Autodesk Inventor part; units mm, degrees
ref_plane "YZ Plane" through (0, 0, 0) normal (1, 0, 0) x (0, 1, 0)
ref_plane "XZ Plane" through (0, 0, 0) normal (0, 1, 0) x (-1, 0, 0)
ref_plane "XY Plane" through (0, 0, 0) normal (0, 0, 1) x (1, 0, 0)
sketch "Sketch1" plane through (0, 0, 0) normal (0, 1, 0) x (-1, 0, 0)
  line L0 (-13, 22.45) -> (13, 22.45)
  line L1 (13, 22.45) -> (13, -22.45)
  line L2 (13, -22.45) -> (-13, -22.45)
  line L3 (-13, -22.45) -> (-13, 22.45)
  line L4 (-13, 22.45) -> (13, -22.45) construction
  line L5 (13, 22.45) -> (-13, -22.45) construction
  point P0 (0, 0)
  dimension "d0" = 26
  dimension "d1" = 44.9
extrude "Extrusion1" add sketch "Sketch1" along normal blind 50
sketch "Sketch2" plane through (-13, 0, 22.45) normal (0, 0, 1) x (1, 0, 0)
  line L0 (0, 0) -> (26, 0)
  line L1 (26, 0) -> (26, 50)
  line L2 (0, 50) -> (26, 50)
  line L3 (0, 0) -> (0, 50)
  line L4 (13, 50) -> (13, 0)
  line L5 (13, 50) -> (7, 50)
  line L6 (26, 50) -> (0, 50)
  line L7 (7, 50) -> (7, 31)
  line L8 (7, 31) -> (19, 31)
  line L9 (19, 31) -> (19, 50)
  line L10 (13, 50) -> (19, 50)
  dimension "d4" = 6
  dimension "d5" = 19
  dimension "d6" = 12
extrude "Extrusion2" cut sketch "Sketch2" against normal blind 50 contours L8 L7 L2 L4 | L4 L2 L9 L8
sketch "Sketch3" plane through (13, 0, 22.45) normal (1, 0, 0) x (0, 0, -1)
  circle A0 centre (7.35, 39.4) radius 1.9
  circle A1 centre (37.55, 39.4) radius 1.9
  line L0 (0, 50) -> (44.9, 50)
  line L1 (22.45, 50) -> (22.45, 0)
  line L2 (44.9, 0) -> (0, 0)
  point P0 (22.45, 25)
  point P1 (3.8014, 50)
  dimension "d9" = 3.8
extrude "Extrusion3" cut sketch "Sketch3" against normal blind 50
sketch "Sketch4" plane through (0, 0, 0) normal (0, -1, 0) x (1, 0, 0)
  circle A0 centre (-8, -17.5) radius 2.5
  circle A1 centre (8, -17.5) radius 2.5
  circle A2 centre (-8, 17.5) radius 2.5
  circle A3 centre (8, 17.5) radius 2.5
  point P0 (0, 0)
extrude "Extrusion4" cut sketch "Sketch4" against normal blind 12
properties part number "housing"
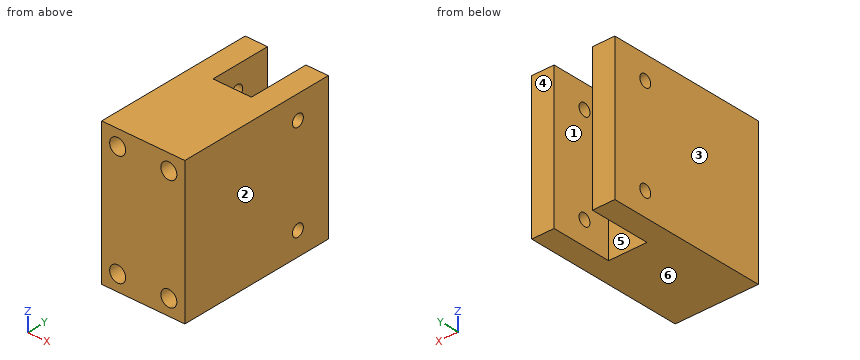
Check sheet for the modelled part. Datum: model origin and axes. Units: mm. Face numbers are marked on the shaded views. A direction names the side the tool comes from. Coordinates: 2 decimals unless noted, no trailing zeros. Write each loop counter-clockwise with the first axis right and the second up, starting at its lowest first coordinate (ties: lowest second). Pieces come first, ordered by that corner, then holes. Notation, with made-up numbers: (18, 74.25) -> (32, 74.25) arc R15 ccw to (32, 95.25) -> close; hole circle Ø3 at (75, -16). An arc over 180 degrees is marked (long way). Use a Markdown table: item, result.
1. Sectioned sample at B-B (x = -8). Enter the section's corners in (y, z).
Reported:
| item | result |
|---|---|
| outline | (0, -22.45) -> (50, -22.45) -> (50, 22.45) -> (0, 22.45) -> (0, 20) -> (12, 20) -> (12, 15) -> (0, 15) -> (0, -15) -> (12, -15) -> (12, -20) -> (0, -20) -> close; hole circle Ø3.8 at (39.4, -15.1); hole circle Ø3.8 at (39.4, 15.1) |
2. Tool access check on the marked faces 5 and 6. Record the directions out of +Z, -Z, +X, -X, +Y, -Y that give a thin tool (end or side, any length) a straight path to the whole face; none if there is none.
Reported:
| item | result |
|---|---|
| face 5 | +Z, -Z, +Y |
| face 6 | -Z, +X, -X, +Y, -Y |
3. Sectioned sample at A-A (y = 39.4). Enter the section's corners in (x, z), plus the area to 3 significant figures.
Reported:
| item | result |
|---|---|
| outline | (-13, -22.45) -> (-6, -22.45) -> (-6, -17) -> (-13, -17) -> close; (-13, -13.2) -> (-6, -13.2) -> (-6, 13.2) -> (-13, 13.2) -> close; (-13, 17) -> (-6, 17) -> (-6, 22.45) -> (-13, 22.45) -> close; (6, -22.45) -> (13, -22.45) -> (13, -17) -> (6, -17) -> close; (6, -13.2) -> (13, -13.2) -> (13, 13.2) -> (6, 13.2) -> close; (6, 17) -> (13, 17) -> (13, 22.45) -> (6, 22.45) -> close |
| area | 522 mm2 |
4. Sectioned sample at C-C (y = 7). Enter the section's corners in (x, z), plus the area to 3 significant figures.
Reported:
| item | result |
|---|---|
| outline | (-13, -22.45) -> (13, -22.45) -> (13, 22.45) -> (-13, 22.45) -> close; hole circle Ø5 at (-8, -17.5); hole circle Ø5 at (-8, 17.5); hole circle Ø5 at (8, -17.5); hole circle Ø5 at (8, 17.5) |
| area | 1,090 mm2 |
5. Release check for a two-part mould opening along X. For the marked faces 1, 2, 3 and 4 record: pulls with the +X half, pulls with the -X half, needs draft (parallel to the pull), parting line crosses it, or undercut.
Reported:
| item | result |
|---|---|
| face 1 | undercut |
| face 2 | pulls with the +X half |
| face 3 | pulls with the -X half |
| face 4 | needs draft |
6. Sectioned sample at D-D (z = -14). Enter the section's corners in (x, y).
Reported:
| item | result |
|---|---|
| outline | (-13, 0) -> (13, 0) -> (13, 37.85) -> (6, 37.85) -> (6, 31) -> (-6, 31) -> (-6, 37.85) -> (-13, 37.85) -> close; (-13, 40.95) -> (-6, 40.95) -> (-6, 50) -> (-13, 50) -> close; (6, 40.95) -> (13, 40.95) -> (13, 50) -> (6, 50) -> close |
7. Go/stop test with flat-tipped pins: pin 1 Ø3.5 at (y, z) = (39.4, 15.1) entering from -X; pin 2 Ø2.5 at (x, z) = (-8.5, 17) entering from -Y; pin 3 Ø1 at (x, z) = (-1, 4) entering from +Y. Record where each tip stops, or that it passes through.
Reported:
| item | result |
|---|---|
| pin 1 | passes through |
| pin 2 | stops at y = 12 |
| pin 3 | stops at y = 31 |
8. Scan lines: line 1 along Z through (x, y) = (8, 5); line 2 along Y through (x, z) = (-9.25, 15.1); line 3 along X through (y, z) = (38, 4). Record each from-to range of solid material in increasing order.
Reported:
| item | result |
|---|---|
| line 1 | z = -22.45 to -20, -15 to 15, 20 to 22.45 |
| line 2 | y = 0 to 37.5, 41.3 to 50 |
| line 3 | x = -13 to -6, 6 to 13 |
